Autodesk Inventor part; units mm, degrees
ref_plane "Work Plane1" through (71.3599, 83, -75) normal (0, -0.9062, -0.4229) x (1, 0, 0)
ref_plane "YZ Plane" through (0, 0, 0) normal (1, 0, 0) x (0, 1, 0)
ref_plane "XZ Plane" through (0, 0, 0) normal (0, 1, 0) x (-1, 0, 0)
sketch "Sketch1" plane through (0, 0, 0) normal (0, 1, 0) x (-1, 0, 0)
  circle A0 centre (0, 0) radius 75
  dimension "d0" = 150
extrude "Extrusion1" add sketch "Sketch1" along normal blind 83
ref_plane "Work Plane1" through (71.3599, 83, -75) normal (0, -0.9062, -0.4229) x (1, 0, 0)
sketch "Sketch4" plane through (71.3599, 83, -75) normal (0, -0.9062, -0.4229) x (1, 0, 0)
  line L0 (-176.8472, 196.5702) -> (33.3097, 196.5702)
  line L1 (33.3097, 196.5702) -> (33.3097, -66.4056)
  line L2 (33.3097, -66.4056) -> (-176.8472, -66.4056)
  line L3 (-176.8472, -66.4056) -> (-176.8472, 196.5702)
  point P0 (-71.3599, 103.0632)
extrude "Extrusion4" cut sketch "Sketch4" against normal blind 80
sketch "Sketch5" plane through (0, 0, 0) normal (0, -1, 0) x (1, 0, 0)
  circle A0 centre (0, 0) radius 75
  line L0 (38, 64.6607) -> (-38, 64.6607)
  line L1 (-38, 64.6607) -> (-38, -55.3393)
  line L2 (-38, -55.3393) -> (38, -55.3393)
  line L3 (38, -55.3393) -> (38, 64.6607)
  dimension "d9" = 76
  dimension "d10" = 120
extrude "Extrusion5" add sketch "Sketch5" against normal blind 188 contours L3 L2 L1 L0
sketch "Sketch6" plane through (38, 17.825, 64.6607) normal (1, 0, 0) x (0, 0, -1)
  circle A0 centre (60, 110.175) radius 60
  line L0 (0, 170.175) -> (120, 170.175)
  line L1 (0, 0) -> (0, 170.175)
  circle A1 centre (60, 110.175) radius 56
  line L2 (0, 110.175) -> (0, 0)
  line L3 (0, 0) -> (139.6607, 65.175)
  circle A2 centre (-18.8653, 40.855) radius 45
  point P0 (64.6607, -17.825)
  point P1 (0, 110.175)
  point P2 (60, 170.175)
  point P3 (0, 81.7096)
  point P4 (0, 0.0004)
  point P5 (14.9341, 70.5636)
  dimension "d13" = 120
  dimension "d20" = 112
  dimension "d32" = 90
extrude "Extrusion6" cut sketch "Sketch6" against normal blind 188 contours A0 L1 L0
sketch "Sketch7" plane through (-38, 73.825, -55.3393) normal (-1, 0, 0) x (0, 0, 1)
  circle A0 centre (60, 54.175) radius 60
  line L0 (0, 0) -> (0, 114.175)
  line L1 (0, 0) -> (0, 114.175)
  line L2 (60, 114.175) -> (0, 114.175)
  line L3 (0, 114.175) -> (60, 114.175)
  line L4 (60, 114.175) -> (0, 114.175)
  circle A1 centre (60, 54.175) radius 56
  circle A2 centre (60, 54.175) radius 25
  point P0 (55.3393, -73.825)
  point P1 (0, 54.175)
  dimension "d16" = 120
  dimension "d23" = 112
  dimension "d26" = 50
extrude "Extrusion7" cut sketch "Sketch7" against normal blind 188 contours A0 L0 L2
extrude "Extrusion8" add sketch "Sketch6" along normal blind 2 contours A1
extrude "Extrusion9" add sketch "Sketch7" along normal blind 2 contours A1 | A2
extrude "Extrusion10" cut sketch "Sketch7" against normal blind 100 contours A2
extrude "Extrusion11" cut sketch "Sketch7" along normal blind 100 contours A2
extrude "Extrusion12" cut sketch "Sketch6" against normal blind 100 contours A2 L1 picked at (2.4551, 28.6667)
extrude "Extrusion13" cut sketch "Sketch6" against normal blind 100 contours A2 L1 A0
The listing builds one solid part. Answer for the finished solid, in the listing's coordinates (mm). A direction names the side the tool comes from. Coordinates: 2 decimals unless noted, no trailing zeros. Order: outer loops, then holes, each group sorted by start corner. A loop starts at its lowest first (then second) coordinate and runs counter-clockwise, first axis right, second up. Notation, with made-up numbers: M -5,26 L 18,26 A15 cw 18,36 Z; hole C 4,89.25 d3. An arc over 180 degrees is marked long. Answer as a JSON object with one key per item and string values. Group by question number.
1. Section D-D on z = -27 is taken. Write down the section's boundary in (x, y), then the cut area to 3 significant figures.
2. Straight lines are drawn through the part: line 1 (Z direction, x = -17.5, y = 128); line 2 (Y direction, x = 39, z = 24); line 3 (X direction, y = 164, z = 50). For each, find the intervals that lie inside material, in ascending order.
3. A tool of negligible diameter and unlimited length cuts with its end or side. For faces 1 (the flat face through (38, 71, -9)), 2 (the flat face through (-38, 71, 0)), 3 (the cylindrical face through (0.532, 48.79, 39.626)), 4 (the cylindrical face through (-0.53, 183.55, 27.34)), 5 (the flat face through (38.539, 55.086, -15.189)), from which of +Z, -Z, +X, -X, +Y, -Y can it reach the whole face along a straight path? Write none if from no direction.
4. Section B-B on y = 123 is taken. Write down the section's boundary in (x, z).
5. Flat-ended cylindrical pins translate along their axes: P1, Ø2, axis at y = 112.5, z = -36, coming from the +X side; P2, Ø1.5, axis at x = 32.5, y = 87, coming from the -Z side; P3, Ø4, axis at y = 152, z = 10.5, coming from the -X side; P4, Ø6, axis at x = -7.5, z = 41, coming from the -Y side. Find the tip coordinate at first contact, or state that the pin passes through.
6. Determine the mould class of faces 6 (the flat face through (-1, 0, 1)), 7 (the flat face through (-0.532, 15.912, 68.754)), 8 (the cylindrical face through (-0.56, 152.787, 1.406)), 9 (the flat face through (-1, 101, -55.339)) for opening direction Y: released by +Y, released by -Y, zero draft, split by the parting line, or undercut.
7. Section A-A on z = -8.5 is taken. Write down the section's boundary in (x, y).
Values follow:
{
 "1": {"outline": "M -69.97,0 L 69.97,0 L 69.97,60.6 L 38,60.6 L 38,81.81 L 40,81.81 L 40,174.19 L 38,174.19 L 38,178.97 L -38,178.97 L -38,174.19 L -40,174.19 L -40,81.81 L -38,81.81 L -38,60.6 L -69.97,60.6 Z", "area": "17,800 mm2"},
 "2": {"line 1": "-55.34 to -20.34, 29.66 to 64.66", "line 2": "0 to 36.8, 75.45 to 112.16, 143.84 to 180.55", "line 3": "-38 to 38"},
 "3": {"face 1": "+X", "face 2": "-X", "face 3": "+Z, +X, -X", "face 4": "+X, -X", "face 5": "none"},
 "4": {"outline": "M -40,-51.12 L -38,-51.12 L -38,-55.34 L 38,-55.34 L 38,-51.12 L 40,-51.12 L 40,-19.83 L -40,-19.83 Z; M -40,29.16 L 40,29.16 L 40,60.44 L 38,60.44 L 38,64.45 L -38,64.45 L -38,60.44 L -40,60.44 Z"},
 "5": {"P1": "x = 40", "P2": "z = -55.34", "P3": "x = -40", "P4": "y = 0"},
 "6": {"face 6": "released by -Y", "face 7": "released by +Y", "face 8": "undercut", "face 9": "zero draft"},
 "7": {"outline": "M -74.52,0 L 74.52,0 L 74.52,51.96 L 38,51.96 L 38,73.57 L 40,73.57 L 40,106.74 L -40,106.74 L -40,73.57 L -38,73.57 L -38,51.96 L -74.52,51.96 Z; M -40,149.26 L 40,149.26 L 40,182.43 L 38,182.43 L 38,186.54 L -38,186.54 L -38,182.43 L -40,182.43 Z"}
}
